Read the model definition and answer for the solid it produces. Units are mm, in the model's axes. A direction names the side the tool comes from. Coordinates: 2 decimals unless noted, no trailing zeros. Write each loop counter-clockwise with the first axis right and the second up, starting at its lowest first coordinate (ties: lowest second). Pieces come first, ordered by that corner, then holes.
Item 1: Straight lines are drawn through the part: probe 1 along X at (y, z) = (707, 0); probe 2 along X at (y, z) = (709.5, 0); probe 3 along X at (y, z) = (746.5, 0). For each, find the intervals that lie inside material, in ascending order.
Item 2: Each of these flat-tipped pins is pushed along its axis until it touches: P1, Ø6, axis at x = 81, y = 842.5, coming from the -Z side; P2, Ø4, axis at x = 83.25, z = 0, coming from the +Y side; P3, Ø10, axis at y = 829.5, z = 4, coming from the -X side. Where does it stop, or does it pass through?
Item 3: A tool of negligible diameter and unlimited length cuts with its end or side. For faces 5 (the face through (102.7, 826.62, 2.55)), 6 (the face through (61.944, 710.158, -0.045)), 7 (the face through (109, 714.497, 0)), 8 (the face through (119.853, 762.387, -0.044)), from which of +Z, -Z, +X, -X, +Y, -Y can it reach the whole face along a straight path? Write none if from no direction.
Item 4: Determine the mould class of faces 1 (the face through (92, 701.797, 0)), 2 (the face through (102.697, 825.774, -2.685)), 3 (the face through (61.84, 717.45, -0.05)), 4 (the face through (81.7, 708.06, 0.34)) for opening direction X: released by +X, released by -X, zero draft, split by the parting line, or undercut.
Item 5: Section B-B (y = 782) is taken. Give the vertices of the cut face in (x, z) (3 decimals).
Item 6: Section A-A (x = 86.5) is taken. Give the vertices of the cut face in (y, z), then the cut area to 3 significant figures.
from build123d import *

# Parameters (mm, degrees)
BOSS_EXTRUDE1_DEPTH      = 9.525
BOSS_EXTRUDE1_DEPTH_BACK = 9.525
CUT_SWEEP2_START         = 153.457157687
CUT_SWEEP2_OUTLINE_W     = 59
CUT_SWEEP2_OUTLINE_H     = 64
CUT_SWEEP2_DEPTH         = 10.542842313
CUT_SWEEP6_START         = 153.457157687
CUT_SWEEP6_OUTLINE_W     = 53
CUT_SWEEP6_OUTLINE_H     = 64
CUT_SWEEP6_DEPTH         = 9.143384714
SKETCH21_W               = 71.62814367
SKETCH21_H               = 75.485551221
CUT_EXTRUDE5_DEPTH       = 47.371
CUT_EXTRUDE6_DEPTH       = 875.211365037
CUT_EXTRUDE6_DEPTH_BACK  = 875.211365037
SKETCH23_R               = 3.175
CUT_EXTRUDE7_DEPTH       = 558.8
CUT_EXTRUDE17_DEPTH      = 875.211365037
CUT_EXTRUDE17_DEPTH_BACK = 875.211365037
SKETCH24_W               = 149.671164142
SKETCH24_H               = 168.486967634
SKETCH24_H_2             = 161.925
SKETCH31_R               = 1.5875
CUT_EXTRUDE18_DEPTH      = 12.7


with BuildPart() as part:
    # Sketch1 → Boss-Extrude1 (new, two sides: drawn at the far end of the back side and taken through both)
    with BuildSketch(Plane.XY.offset(-BOSS_EXTRUDE1_DEPTH_BACK)):
        Polygon((57.217766507, 219.836565958), (134.681996719, 219.836565958), (125.140068317, 803.55209701), (88.830980485, 863.721914098), (57.217766507, 807.103985498), align=None)
    extrude(amount=BOSS_EXTRUDE1_DEPTH + BOSS_EXTRUDE1_DEPTH_BACK)

    # Cut-Sweep1: sweep along a path in Sketch4
    with BuildLine(Plane.XY.offset(9.525)) as cut_sweep1_path:
        Line((95.949881613, 219.836565958), (88.830980485, 863.721914098))
    # Sketch2 → Cut-Sweep1 (sweep, cut)
    with BuildSketch(Plane.XZ.offset(-219.836565958)):
        Polygon((95.949881613, 9.525), (134.681996719, 0), (134.681996719, 9.525), align=None)
    sweep(path=cut_sweep1_path.line, mode=Mode.SUBTRACT)

    # Cut-Sweep2: read off the stored shape, not the designer's step
    # Cut-Sweep2 outline → Cut-Sweep2 (cut)
    with BuildSketch(Plane(origin=(0, 0, 0), x_dir=(0.9721406430200956, -0.0370263288920756, -0.23145544097568965), z_dir=(0.2343983152423991, 0.15356253367517805, 0.9599354030677193)).offset(CUT_SWEEP2_START)):
        with Locations((63.5, 822)):
            Rectangle(CUT_SWEEP2_OUTLINE_W, CUT_SWEEP2_OUTLINE_H)
    extrude(amount=CUT_SWEEP2_DEPTH, mode=Mode.SUBTRACT)

    # Cut-Sweep3: sweep along a path in Sketch8
    with BuildLine(Plane.XY.offset(9.525)) as cut_sweep3_path:
        Line((95.949881613, 219.836565958), (88.830980485, 863.721914098))
    # Sketch7 → Cut-Sweep3 (sweep, cut)
    with BuildSketch(Plane.XZ.offset(-219.836565958)):
        Polygon((95.949881613, 9.525), (57.217766507, 0), (57.217766507, 9.525), align=None)
    sweep(path=cut_sweep3_path.line, mode=Mode.SUBTRACT)

    # Cut-Sweep4: sweep along a path in Sketch10
    with BuildLine(Plane(origin=(3.4015871, 0.0376085, -13.832090615), x_dir=(0.9710677735095292, -0.0006492893666849942, 0.23880317768941897), z_dir=(-0.23880406037428656, -0.002640256529482778, 0.9710641841784778))) as cut_sweep4_path:
        Line((55.419591582, 807.105343631), (88.664251397, 803.18099011))
    # Sketch9 → Cut-Sweep4 (sweep, cut)
    with BuildSketch(Plane(origin=(98.36840601, 1.087577095, 0), x_dir=(0, 0, 1), z_dir=(-0.9999388862366849, -0.011055486951654862, 0))):
        Polygon((9.525, 802.119504525), (27.927952665, 862.687059056), (0, 862.687059056), align=None)
    sweep(path=cut_sweep4_path.line, mode=Mode.SUBTRACT)

    # Cut-Sweep5: sweep along a path in Sketch12
    with BuildLine(Plane(origin=(0, 0, -9.525), x_dir=(-1, 0, 0), z_dir=(0, 0, -1))) as cut_sweep5_path:
        Line((-88.830980485, 863.721914098), (-95.949881613, 219.836565958))
    # Sketch11 → Cut-Sweep5 (sweep, cut)
    with BuildSketch(Plane.XZ.offset(-219.836565958)):
        Polygon((95.949881613, -9.525), (134.681996719, 0), (134.681996719, -15.883536915), (57.217766507, -15.883536915), (57.217766507, 0), align=None)
    sweep(path=cut_sweep5_path.line, mode=Mode.SUBTRACT)

    # Cut-Sweep6: read off the stored shape, not the designer's step
    # Cut-Sweep6 outline → Cut-Sweep6 (cut)
    with BuildSketch(Plane(origin=(0, 0, 0), x_dir=(0.9721406430200958, -0.03702632889207545, 0.2314554409756887), z_dir=(0.23439831524239813, 0.1535625336751781, -0.9599354030677195)).offset(CUT_SWEEP6_START)):
        with Locations((66.5, -822)):
            Rectangle(CUT_SWEEP6_OUTLINE_W, CUT_SWEEP6_OUTLINE_H)
    extrude(amount=CUT_SWEEP6_DEPTH, mode=Mode.SUBTRACT)

    # Sketch21 → Cut-Extrude5 (cut)
    with BuildSketch(Plane(origin=(-23.933102236, 16.341018935, -105.585382191), x_dir=(-0.9758175121644082, -0.033431767496308724, 0.2160150454837301), z_dir=(-0.2185867858615091, 0.14924646088248067, -0.9643367207364807))):
        with Locations((-95.99768501, 822.261491576)):
            Rectangle(SKETCH21_W, SKETCH21_H)
    extrude(amount=CUT_EXTRUDE5_DEPTH, mode=Mode.SUBTRACT)

    # Sketch22 → Cut-Extrude6 (cut, two sides: drawn at the far end of the back side and taken through both)
    with BuildSketch(Plane.XY.offset(-CUT_EXTRUDE6_DEPTH_BACK)):
        with BuildLine():
            Line((57.217766507, 737.561994928), (64.475710809, 732.15618288))
            ThreePointArc((64.475710809, 732.15618288), (64.859122479, 731.376710767), (64.450428737, 730.610192203))
            Line((64.450428737, 730.610192203), (57.217766507, 725.582342683))
            Line((57.217766507, 725.582342683), (57.217766507, 737.561994928))
        make_face()
        with BuildLine():
            Line((57.217766507, 722.071065301), (64.863611969, 714.425219839))
            ThreePointArc((64.863611969, 714.425219839), (65.14259276, 713.751700629), (64.863611969, 713.07818142))
            Line((64.863611969, 713.07818142), (57.217766507, 705.432335958))
            Line((57.217766507, 705.432335958), (57.217766507, 722.071065301))
        make_face()
        with BuildLine():
            Line((125.746024678, 766.483474766), (115.991696873, 759.702666979))
            ThreePointArc((115.991696873, 759.702666979), (115.583003131, 758.936148415), (115.966414801, 758.156676302))
            Line((115.966414801, 758.156676302), (126.004357543, 750.680284978))
            Line((126.004357543, 750.680284978), (125.746024678, 766.483474766))
        make_face()
        with BuildLine():
            Line((130.504368952, 475.397717553), (120.864153688, 462.45458434))
            ThreePointArc((120.864153688, 462.45458434), (120.675678689, 461.901197798), (120.845958337, 461.341944429))
            Line((120.845958337, 461.341944429), (130.972260191, 446.775056406))
            Line((130.972260191, 446.775056406), (130.504368952, 475.397717553))
        make_face()
        with BuildLine():
            Line((57.217766507, 423.998589411), (65.145848829, 412.59388421))
            ThreePointArc((65.145848829, 412.59388421), (65.316128476, 412.03463084), (65.127653478, 411.481244299))
            Line((65.127653478, 411.481244299), (57.217766507, 400.861282196))
            Line((57.217766507, 400.861282196), (57.217766507, 423.998589411))
        make_face()
    extrude(amount=CUT_EXTRUDE6_DEPTH + CUT_EXTRUDE6_DEPTH_BACK, mode=Mode.SUBTRACT)

    # Sketch23 → Cut-Extrude7 (cut)
    with BuildSketch(Plane.XZ.offset(-219.836565958)):
        with Locations(Location((95.949881613, 0, 0), (0, 0, 270))):
            Circle(SKETCH23_R)
    extrude(amount=-CUT_EXTRUDE7_DEPTH, mode=Mode.SUBTRACT)

    # Sketch24 → Cut-Extrude17 (cut, two sides: drawn at the far end of the back side and taken through both)
    with BuildSketch(Plane.XY.offset(-CUT_EXTRUDE17_DEPTH_BACK)):
        with Locations((94.66698592, 293.703430281)):
            Rectangle(SKETCH24_W, SKETCH24_H)
        with Locations((94.66698592, 458.909414098)):
            Rectangle(SKETCH24_W, SKETCH24_H_2)
        with Locations((94.66698592, 620.834414098)):
            Rectangle(SKETCH24_W, SKETCH24_H_2)
    extrude(amount=CUT_EXTRUDE17_DEPTH + CUT_EXTRUDE17_DEPTH_BACK, mode=Mode.SUBTRACT)

    # Sketch31 → Cut-Extrude18 (cut)
    with BuildSketch(Plane.XZ.offset(-701.796914098)):
        with Locations(Location((83.249881613, 0, 0), (0, 0, 270))):
            Circle(SKETCH31_R)
        with Locations(Location((108.649881613, 0, 0), (0, 0, 270))):
            Circle(SKETCH31_R)
    extrude(amount=-CUT_EXTRUDE18_DEPTH, mode=Mode.SUBTRACT)


solid = part.part
Established:
1. probe 1: x = 58.79 to 81.66, 84.84 to 92.77, 99.12 to 107.06, 110.24 to 126.72
1. probe 2: x = 61.29 to 81.66, 84.84 to 92.77, 99.12 to 107.06, 110.24 to 126.68
1. probe 3: x = 57.22 to 92.77, 99.12 to 126.07
2. P1: stops at z = -2.33
2. P2: stops at y = 857.31
2. P3: stops at x = 67.46
3. face 5: +Z, +X, +Y
3. face 6: +Z, -Z, -X
3. face 7: -Y
3. face 8: +Z, -Z, +X
4. face 1: zero draft
4. face 2: released by +X
4. face 3: released by -X
4. face 4: undercut
5. outline: (57.218, -1.528) - (89.735, -9.525) - (125.492, -0.731) - (125.492, 0.731) - (89.735, 9.525) - (57.218, 1.528) - close
6. outline: (701.8, -8.51) - (803.52, -8.79) - (859.55, -0.12) - (859.55, 0.12) - (803.52, 8.79) - (701.8, 8.51) - close
6. area: 2,260 mm2
